from build123d import *

# Parameters (mm, degrees)
F0_R          = 3.95
F1_DEPTH      = 35.86
F1_DEPTH_BACK = 35.86
F2_R          = 2.575
F3_DEPTH      = 7
F4_R          = 2.575
F5_DEPTH      = 7


with BuildPart() as f1:
    # F0 (on Front) → F1 (new body, two sides)
    with BuildSketch(Plane.XZ) as f1_sk:
        Circle(F0_R)
    extrude(amount=F1_DEPTH)
    extrude(f1_sk.sketch, amount=-F1_DEPTH_BACK)

    # F2 (on face) → F3 (join)
    with BuildSketch(Plane(origin=(0, 35.86, 0), x_dir=(-1, 0, 0), z_dir=(0, 1, 0))):
        Circle(F2_R)
    extrude(amount=F3_DEPTH)

    # F4 (on face) → F5 (join)
    with BuildSketch(Plane.XZ.offset(35.86)):
        Circle(F4_R)
    extrude(amount=F5_DEPTH)


solid = f1.part
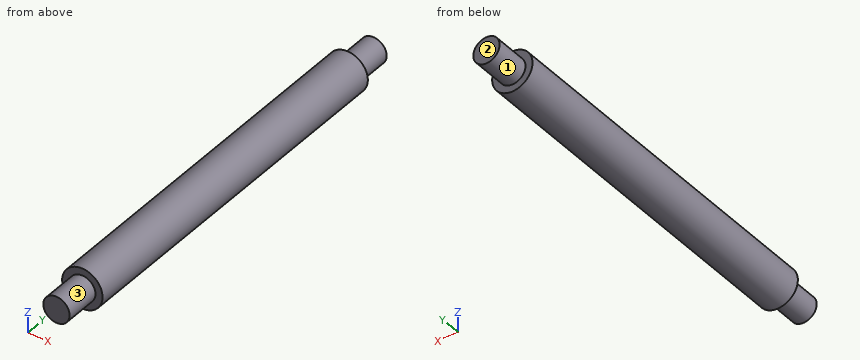
Can you work these out from the model? Positions are in its coordinate system, mm. Face numbers are marked on the shaded views. A direction names the side the tool comes from. Coordinates: 2 decimals unless noted, no trailing zeros. Loops run counter-clockwise (first coordinate to the right, second up) from the corner with the lowest first, then second, coordinate; pieces in that order, holes last. Notation, with made-up numbers: M 79,71.25 L 128,71.25 A13 cw 128,82.25 Z; hole C 81.25,51.25 d11. An arc over 180 degrees is marked long. Return JSON: item names as keys, results as strings. Group by question number.
Item 1: On a 3-axis mill with a long thin cutter (end or side, diameter ignored), from which of +Z, -Z, +X, -X, +Y, -Y can I reach the whole of each face in a straight line? I mean the marked faces 1, 2 and 3. Say none if no direction works.
Item 2: If I drill on L1, parallel to Z at x = 0.25, y = 17; L2, parallel to Z at x = 3, y = -27; L3, parallel to Y at x = 1.25, z = -3.25, over which ranges is the centre line in solid material (lowest first)? Write a range as from..to.
Item 3: I'm going to push flat-ended pins straight in: pin 1 Ø3 at (x, y) = (-1.5, -34) entering from +Z; pin 2 Ø1.5 at (y, z) = (-24, -2.5) entering from +X. Where does each tip first touch, or does it pass through?
Item 4: Imagine slicing it at A-A (z = 0). Please give me the cut outline in (x, y) (3 decimals), and give its area (3 significant figures).
Item 5: Imagine slicing it at C-C (y = -4). Please give me the cut outline in (x, z), and give its area (3 significant figures).
Item 6: Imagine slicing it at B-B (x = 0). Please give me the cut outline in (y, z) (3 decimals).
Verdict:
{
 "1": {"face 1": "+Y", "face 2": "+Z, -Z, +X, -X, +Y", "face 3": "-Y"},
 "2": {"L1": "z = -3.94..3.94", "L2": "z = -2.57..2.57", "L3": "y = -35.86..35.86"},
 "3": {"pin 1": "stops at z = 3.95", "pin 2": "stops at x = 3.54"},
 "4": {"outline": "M -3.95,-35.86 L -2.575,-35.86 L -2.575,-42.86 L 2.575,-42.86 L 2.575,-35.86 L 3.95,-35.86 L 3.95,35.86 L 2.575,35.86 L 2.575,42.86 L -2.575,42.86 L -2.575,35.86 L -3.95,35.86 Z", "area": "639 mm^2"},
 "5": {"outline": "C 0,0 d7.9", "area": "49.0 mm^2"},
 "6": {"outline": "M -42.86,-2.575 L -35.86,-2.575 L -35.86,-3.95 L 35.86,-3.95 L 35.86,-2.575 L 42.86,-2.575 L 42.86,2.575 L 35.86,2.575 L 35.86,3.95 L -35.86,3.95 L -35.86,2.575 L -42.86,2.575 Z"}
}
